Geometry check sheet. Reference: the model listing, model coordinates, mm. Face numbers are marked on the shaded views. Give positions to 0.01 mm unless a question says otherwise; leave off trailing zeros. Write each loop counter-clockwise with the first axis right and the second up, starting at its lowest first coordinate (ties: lowest second). Pieces come first, ordered by that corner, then holes. Notation, with made-up numbers: (67, -5) -> (95, -5) arc R13 ccw to (95, 20) -> close; hole circle Ø8 at (-22, -32.5). An arc over 180 degrees is marked (long way). Write item = value, one per line. Start each with the question number.
1. Cross-section at A-A, the plane z = 81. Record the cut outline in (x, y).
2. Mould release check, pull along Y, two halves, no side actions. Record for the marked faces 1 and 2: pulls with the +Y half, pulls with the -Y half, needs draft (parallel to the pull), parting line crosses it, or undercut.
3. Thickness scan on line 1 along Y through (x, z) = (0, 171); line 2 along Z through (x, y) = (5, 1.5) (3 decimals); line 3 along Y through (x, z) = (4, 131). Record the ranges inside material, lowest first.
4. Cross-section at B-B, the plane x = -14. Record the cut outline in (y, z) (3 decimals), plus the area to 3 significant figures.
5. Depth check by flat-ended pin: P1, Ø1, axis at x = -4.5, y = -12, coming from the +Z side; P2, Ø12, axis at x = -7.5, z = 262, coming from the +Y side; P3, Ø16.5, axis at x = 9, y = -11, coming from the +Z side. Enter the tip coordinate at first touch or a pass-through.
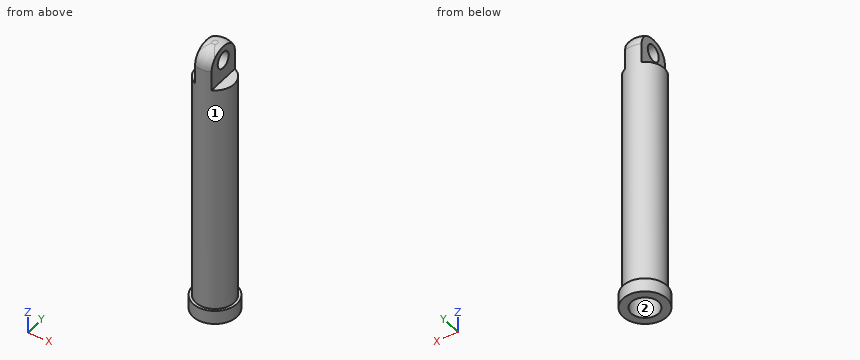
```python
from build123d import *

# Parameters (mm, degrees)
SKETCH_1_R          = 70
EXTRUDE_2_DEPTH     = 1150
CUT_EXTRUDE_START   = -130
CUT_EXTRUDE_1_DEPTH = 130
SKETCH_3_R          = 30
CUT_EXTRUDE_2_DEPTH = 130
FILLET_1_R          = 60
SKETCH_4_R          = 50
CUT_EXTRUDE_3_DEPTH = 977
SKETCH_5_R          = 79.849645552
CUT_EXTRUDE_4_DEPTH = 100
SKETCH_6_R          = 77.974086693
CUT_EXTRUDE_5_DEPTH = 30
SKETCH_7_R          = 80
SKETCH_7_R_2        = 70
EXTRUDE_4_DEPTH     = 50
SCALE_1_SCALE       = 0.345


with BuildPart() as part:
    # 草图1 → 凸台-拉伸2 (new body)
    with BuildSketch(Plane.XY):
        Circle(SKETCH_1_R)
    extrude(amount=EXTRUDE_2_DEPTH)

    # 草图2 → 切除-拉伸1 (cut)
    with BuildSketch(Plane.XY.offset(1150).offset(CUT_EXTRUDE_START)):
        with BuildLine():
            ThreePointArc((70, 0), (59.160797831, 37.416573868), (30, 63.245553203))
            Line((30, 63.245553203), (30, -63.245553203))
            ThreePointArc((30, -63.245553203), (59.160797831, -37.416573868), (70, 0))
        make_face()
        with BuildLine():
            Line((-30, -63.245553203), (-30, 63.245553203))
            ThreePointArc((-30, 63.245553203), (-70, 0), (-30, -63.245553203))
        make_face()
    extrude(amount=CUT_EXTRUDE_1_DEPTH, mode=Mode.SUBTRACT)

    # 草图3 → 切除-拉伸2 (cut)
    with BuildSketch(Plane(origin=(30, 0, 0), x_dir=(0, 0, -1), z_dir=(1, 0, 0))):
        with Locations((-1095, 0)):
            Circle(SKETCH_3_R)
    extrude(amount=-CUT_EXTRUDE_2_DEPTH, mode=Mode.SUBTRACT)

    # 圆角1
    # the kernel refuses this fillet: 60 mm, written as the material it takes off along each edge
    with BuildSketch(Plane(origin=(0, 0, 1150), x_dir=(0.527411317590309, -0.8496100882626421, 0), z_dir=(-0.8496100882626421, -0.527411317590309, 0))) as fillet_1_piece_1:
        with BuildLine():
            CenterArc((70 - FILLET_1_R, -FILLET_1_R), FILLET_1_R, 0, 90)
            Line((70 - FILLET_1_R, 0), (70, 0))
            Line((70, 0), (70, -FILLET_1_R))
        make_face()
    revolve(axis=Axis((0, 0, 1150), (0, 0, 1)), revolution_arc=296.338571462, mode=Mode.SUBTRACT)
    with BuildSketch(Plane(origin=(0, 0, 1150), x_dir=(-0.527411317590308, 0.8496100882626425, 0), z_dir=(0.8496100882626425, 0.527411317590308, 0))) as fillet_1_piece_2:
        with BuildLine():
            CenterArc((70 - FILLET_1_R, -FILLET_1_R), FILLET_1_R, 0, 90)
            Line((70 - FILLET_1_R, 0), (70, 0))
            Line((70, 0), (70, -FILLET_1_R))
        make_face()
    revolve(axis=Axis((0, 0, 1150), (0, 0, 1)), revolution_arc=296.338571462, mode=Mode.SUBTRACT)

    # 草图4 → 切除-拉伸3 (cut)
    with BuildSketch(Plane(origin=(0, 0, 0), x_dir=(-1, 0, 0), z_dir=(0, 0, -1))):
        Circle(SKETCH_4_R)
    extrude(amount=-CUT_EXTRUDE_3_DEPTH, mode=Mode.SUBTRACT)

    # 草图5 → 切除-拉伸4 (cut)
    with BuildSketch(Plane(origin=(0, 0, 0), x_dir=(-1, 0, 0), z_dir=(0, 0, -1))):
        Circle(SKETCH_5_R)
    extrude(amount=-CUT_EXTRUDE_4_DEPTH, mode=Mode.SUBTRACT)

    # 草图6 → 切除-拉伸5 (cut)
    with BuildSketch(Plane(origin=(0, 0, 100), x_dir=(-1, 0, 0), z_dir=(0, 0, -1))):
        Circle(SKETCH_6_R)
    extrude(amount=-CUT_EXTRUDE_5_DEPTH, mode=Mode.SUBTRACT)

    # 草图7 → 凸台-拉伸4 (add)
    with BuildSketch(Plane(origin=(0, 0, 130), x_dir=(-1, 0, 0), z_dir=(0, 0, -1))):
        Circle(SKETCH_7_R)
        Circle(SKETCH_7_R_2, mode=Mode.SUBTRACT)
    extrude(amount=-EXTRUDE_4_DEPTH)


with BuildPart() as part_1:
    # 缩放比例1: scaled about (0, 0, 0)
    add(part.part.scale(SCALE_1_SCALE))


solid = part_1.part
```
Answers:
q1.outline = circle Ø48.3 at (0, 0); hole circle Ø34.5 at (0, 0)
q2.face_1 = parting line crosses it
q2.face_2 = undercut
q3.line_1 = -24.15 to -17.25, 17.25 to 24.15
q3.line_2 = 337.065 to 367.534, 388.016 to 396.674
q3.line_3 = -23.82 to -16.78, 16.78 to 23.82
q4.outline = (-23.786, 44.85) -> (-10.078, 44.85) -> (-10.078, 337.065) -> (10.078, 337.065) -> (10.078, 44.85) -> (23.786, 44.85) -> (23.786, 62.1) -> (19.678, 62.1) -> (19.678, 351.9) -> (-19.678, 351.9) -> (-19.678, 62.1) -> (-23.786, 62.1) -> close
q4.area = 6,340 mm^2
q5.P1 = 394.76
q5.P2 = 24.1
q5.P3 = 396.6
